Part model, mm, in its own coordinate system. A direction names the side the tool comes from. Coordinates: 2 decimals unless noted, no trailing zeros. Write each loop counter-clockwise with the first axis right and the second up, starting at its lowest first coordinate (ties: lowest second). Pieces come first, ordered by that corner, then holes. Notation, with made-up numbers: M -38,-14.75 L 6,-14.75 A19 cw 6,-2.75 Z; hole C -37.75,39 d5. An arc over 180 degrees is marked long. Use a Markdown table: item, result. Add a question column.
Q1. Mould opens along X. For faces 1 (the flat face through (66, 0, 61.925)), 2 (the flat face through (-41.275, -1, 0)), 3 (the cylindrical face through (46.958, -0.178, 41.215)) say: released by +X, released by -X, zero draft, split by the parting line, or undercut.
Q2. Wall check: L1, parallel to Y at x = 34, z = 17; L2, parallel to X at y = 35, z = 2.5 (3 decimals); L3, parallel to Z at x = 31, y = 45.5 (3 decimals). Give the ranges that are in metal, low to high. Write a range as from..to.
Q3. Tool access for faces 4 (the flat face through (23, 12.7, 40)), 5 (the cylindrical face through (62.67, -0.18, 43.93)), 6 (the flat face through (41.275, -1, 1)), 7 (the flat face through (1, -38, 9.525)): list every direction of +Z, -Z, +X, -X, +Y, -Y with a clear straight run to the whole face (end or side of a thin tool).
Q4. Pin check, flat tips, straight feed: pin 1 Ø2 at (y, z) = (6.5, 40) entering from -X; pin 2 Ø23 at (x, y) = (76, 2) entering from -Z; pin 3 Ø2 at (y, z) = (2.5, 18) entering from -X. Stop position of each tip, or through.
Q5. Slice it at B-B on x = 68. Write the cut outline in (y, z), then the cut area to 3 significant figures.
Q6. Slice it at A-A on z = 1.5. Write the cut outline in (x, y) (3 decimals), then the cut area to 3 significant figures.
from build123d import *

# Parameters (mm, degrees)
F1_DEPTH = 63.5
F2_DEPTH = 12.7
F3_DEPTH = 12.7


with BuildPart() as f1:
    # F0 (on Front) → F1 (new body, symmetric)
    with BuildSketch(Plane.XZ):
        Polygon((-41.275, 9.525), (-41.275, -9.525), (41.275, -9.525), (41.275, 9.525), (22.225, 9.525), align=None)
    extrude(amount=F1_DEPTH, both=True)

    # F0 (on Front) → F2 (join, symmetric)
    with BuildSketch(Plane.XZ):
        with BuildLine():
            Line((22.225, 9.525), (41.275, 9.525))
            Line((41.275, 9.525), (41.275, 29.043647))
            ThreePointArc((41.275, 29.043647), (47.109768, 41.340369), (60.325, 44.597907))
            Line((60.325, 44.597907), (60.325, 61.9252))
            Line((60.325, 61.9252), (45.378887, 61.9252))
            ThreePointArc((45.378887, 61.9252), (28.59425, 49.151475), (22.225, 29.043647))
            Line((22.225, 29.043647), (22.225, 9.525))
        make_face()
        with BuildLine():
            Line((85.725, 61.9252), (60.325, 61.9252))
            Line((60.325, 61.9252), (60.325, 44.597907))
            ThreePointArc((60.325, 44.597907), (62.700375, 43.916743), (64.941262, 42.8752))
            Line((64.941262, 42.8752), (85.725, 42.8752))
            Line((85.725, 42.8752), (85.725, 61.9252))
        make_face()
    extrude(amount=F2_DEPTH, both=True)

    # F0 (on Front) → F3 (join, symmetric)
    with BuildSketch(Plane.XZ):
        with BuildLine():
            add(Edge.make_bspline(
                [(-41.275, 9.525), (-40.837802, 41.657459), (-14.82299, 70.037253), (45.378887, 61.9252)],
                knots=[0, 0, 0, 0, 101.265379, 101.265379, 101.265379, 101.265379], degree=3))
            Line((-41.275, 9.525), (22.225, 9.525))
            Line((22.225, 9.525), (22.225, 29.043647))
            ThreePointArc((22.225, 29.043647), (28.59425, 49.151475), (45.378887, 61.9252))
        make_face()
    extrude(amount=F3_DEPTH, both=True)


solid = f1.part
Recorded:
| question | item | result |
|---|---|---|
| 1 | face 1 | zero draft |
| 1 | face 2 | released by -X |
| 1 | face 3 | undercut |
| 2 | L1 | -12.7..12.7 |
| 2 | L2 | -41.275..41.275 |
| 2 | L3 | -9.525..9.525 |
| 3 | face 4 | +Z, +X, -X, +Y |
| 3 | face 5 | -Z, +Y, -Y |
| 3 | face 6 | -Z, +X, +Y, -Y |
| 3 | face 7 | +Z, +X, -X, -Y |
| 4 | pin 1 | x = -32.13 |
| 4 | pin 2 | z = 42.88 |
| 4 | pin 3 | x = -40.7 |
| 5 | outline | M -12.7,42.88 L 12.7,42.88 L 12.7,61.93 L -12.7,61.93 Z |
| 5 | area | 484 mm² |
| 6 | outline | M -41.275,-63.5 L 41.275,-63.5 L 41.275,63.5 L -41.275,63.5 Z |
| 6 | area | 10,500 mm² |
